Check sheet for the drawn part. Datum: minimum x, y, z corner. Units: mm. Give positions to 0.01 mm unless a question says otherwise; leave off trailing zeros. Order: outer loops, then holes, each group sorted by start corner. A loop starts at its lowest first (then second) coordinate and runs counter-clockwise, first axis right, second up.
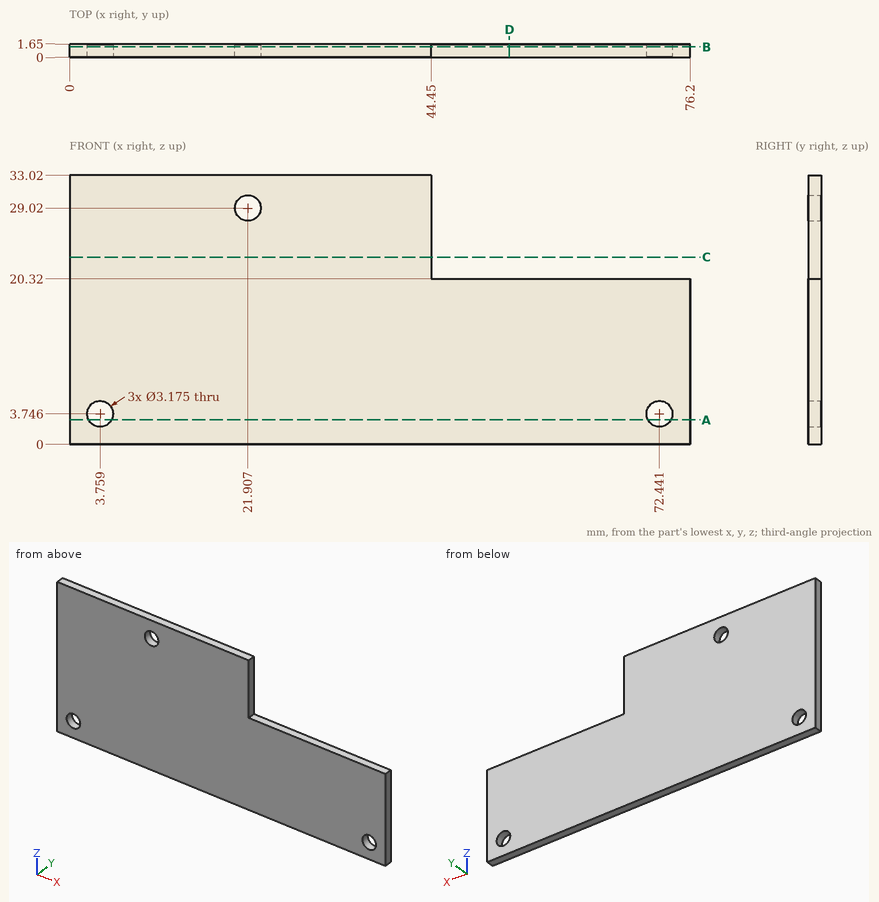
Item 1: Sectioned sample at D-D (x = 54). Enter the section's corners in (y, z).
Reported:
outline: (0, 0) - (1.65, 0) - (1.65, 20.32) - (0, 20.32) - close
Item 2: Gauge pin test, flat ends, axial feed: pin 1 (0.5 mm diameter, centred on y = 1, z = 25.5, fed in from +X); pin 2 (0.5 mm diameter, centred on x = 59, y = 0.5, fed in from +Z). Record the tip position at first contact, or that the pin passes through.
Reported:
pin 1: stops at x = 44.45
pin 2: stops at z = 20.32
Item 3: Sectioned sample at B-B (y = 1.3). Give the number of separate pieces and of enclosed holes in the cut face, and give its area (3 significant figures).
Reported:
separate pieces: 1
enclosed holes: 3
area: 2,090 mm2
Item 4: Sectioned sample at A-A (z = 3). Enter the section's corners in (x, y).
Reported:
outline: (0, 0) - (2.36, 0) - (2.36, 1.65) - (0, 1.65) - close; (5.16, 0) - (71.04, 0) - (71.04, 1.65) - (5.16, 1.65) - close; (73.84, 0) - (76.2, 0) - (76.2, 1.65) - (73.84, 1.65) - close
Item 5: Sectioned sample at C-C (z = 23). Enter the section's corners in (x, y).
Reported:
outline: (0, 0) - (44.45, 0) - (44.45, 1.65) - (0, 1.65) - close
Item 6: Scan lines: L1, parallel to X at y = 1.5, z = 3.5; L2, parallel to X at y = 0.15, z = 5 (1 decimal); L3, parallel to Z at x = 61, y = 1.2. Record each from-to range of solid material in increasing order.
Reported:
L1: x = 0 to 2.19, 5.33 to 70.87, 74.01 to 76.2
L2: x = 0 to 2.8, 4.7 to 71.5, 73.4 to 76.2
L3: z = 0 to 20.32
